Autodesk Inventor part; units mm, degrees
ref_plane "YZ Plane" through (0, 0, 0) normal (1, 0, 0) x (0, 1, 0)
ref_plane "XZ Plane" through (0, 0, 0) normal (0, 1, 0) x (-1, 0, 0)
ref_plane "XY Plane" through (0, 0, 0) normal (0, 0, 1) x (1, 0, 0)
sketch "Sketch1" plane through (0, 0, 0) normal (0, 1, 0) x (-1, 0, 0)
  line L0 (2.0677, 2.6131) -> (-3.5538, 2.6131)
  line L1 (-3.5538, 2.6131) -> (-3.5538, -3.0084)
  line L2 (-3.5538, -3.0084) -> (2.0677, -3.0084)
  line L3 (2.0677, -3.0084) -> (2.0677, 2.6131)
  circle A0 centre (-0.743, -0.1977) radius 3.975
  point P0 (0, 0)
  dimension "d0" = 7.95
extrude "Extrusion1" add sketch "Sketch1" along normal mid plane 50
extrude "Extrusion2" add sketch "Sketch1" along normal mid plane 70 contours L3 L2 L1 L0
hole "Hole1" at (0.743, -35, -0.1977) direction (0, 1, 0) diameter 3 end through all
properties part number "crankshaft_bearing_mounts"
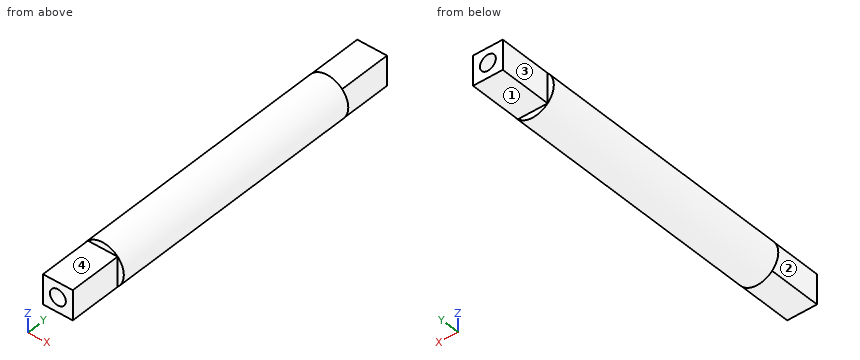
Can you work these out from the model? Positions are in its coordinate system, mm. Face numbers are marked on the shaded views. A direction names the side the tool comes from. Give positions to 0.01 mm unless a question says otherwise; leave off trailing zeros. Order: outer loops, then holes, each group sorted by start corner. A loop starts at its lowest first (then second) coordinate and runs counter-clockwise, first axis right, second up. Notation, with made-up numbers: (28.5, -6) - (66.5, -6) arc R21 cw to (66.5, 5) - close; hole circle Ø10 at (55.25, 51). An arc over 180 degrees is marked (long way). Use a Markdown table: item, result. Add a question column.
Q1. If we section it at A-A on z = 0.5: Write out the boundary of the cut face in (x, y), plus the area to 3 significant figures.
Q2. On a 3-axis mill with a long thin cutter (end or side, diameter ignored), from which of +Z, -Z, +X, -X, +Y, -Y can I reach the whole of each face in a straight line? I mean the marked faces 1, 2, 3 and 4. Say none if no direction works.
Q3. I'm going to push flat-ended pins straight in: pin 1 (4.5 mm diameter, centred on x = 0.5, y = 27.5, fed in from -Z); pin 2 (4.5 mm diameter, centred on y = 31, z = 1, fed in from +X); pin 3 (0.6 mm diameter, centred on x = 0.5, z = -3.5, fed in from -Y). Where does each tip first touch, or does it pass through?
Q4. If we section it at C-C on x = -1.5: Write out the boundary of the cut face in (y, z).
Q5. If we section it at D-D on y = 18: Write out the boundary of the cut face in (x, z) (3 decimals), plus the area to 3 significant figures.
Q6. Please list where these lines run through material, in increasing order: line 1 along X through (y, z) = (-5, 0); line 2 along Y through (x, z) = (3.75, -0.25); line 3 along Z through (x, y) = (1.75, 0.5).
Q7. If we section it at B-B on y = -26: Write out the boundary of the cut face in (x, z).
Answers follow:
| question | item | result |
|---|---|---|
| 1 | outline | (-3.17, -25) - (-2.07, -25) - (-2.07, -35) - (-0.58, -35) - (-0.58, 35) - (-2.07, 35) - (-2.07, 25) - (-3.17, 25) - close; (2.07, -35) - (3.55, -35) - (3.55, -25) - (4.66, -25) - (4.66, 25) - (3.55, 25) - (3.55, 35) - (2.07, 35) - close |
| 1 | area | 318 mm^2 |
| 2 | face 1 | -Z, +X, -X, +Y |
| 2 | face 2 | +Z, -Z, -X, -Y |
| 2 | face 3 | +Z, -Z, -X, +Y |
| 2 | face 4 | +Z, +X, -X, -Y |
| 3 | pin 1 | stops at z = -3.01 |
| 3 | pin 2 | stops at x = 3.55 |
| 3 | pin 3 | stops at y = -25 |
| 4 | outline | (-35, -3.01) - (-25, -3.01) - (-25, -3.48) - (25, -3.48) - (25, -3.01) - (35, -3.01) - (35, 2.61) - (25, 2.61) - (25, 3.08) - (-25, 3.08) - (-25, 2.61) - (-35, 2.61) - close |
| 5 | outline | circle Ø7.95 at (0.743, -0.198); hole circle Ø3 at (0.743, -0.198) |
| 5 | area | 42.6 mm^2 |
| 6 | line 1 | x = -3.23 to -0.74, 2.23 to 4.71 |
| 6 | line 2 | y = -25 to 25 |
| 6 | line 3 | z = -4.04 to -1.31, 0.91 to 3.65 |
| 7 | outline | (-2.07, -3.01) - (3.55, -3.01) - (3.55, 2.61) - (-2.07, 2.61) - close; hole circle Ø3 at (0.74, -0.2) |
